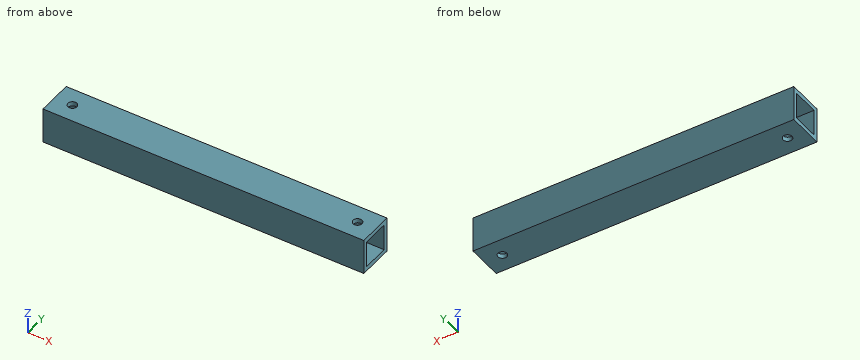
```python
from build123d import *

# Parameters (mm, degrees)
SKETCH1_W           = 228.6
SKETCH1_H           = 25.4
BOSS_EXTRUDE1_DEPTH = 25.4
SKETCH2_W           = 9.525
SKETCH2_H           = 19.040717284
CUT_EXTRUDE1_DEPTH  = 508
SKETCH4_R           = 3.175
CUT_EXTRUDE3_DEPTH  = 508


with BuildPart() as part:
    # Sketch1 → Boss-Extrude1 (new body)
    with BuildSketch(Plane.XY):
        Rectangle(SKETCH1_W, SKETCH1_H)
    extrude(amount=BOSS_EXTRUDE1_DEPTH)

    # Sketch2 → Cut-Extrude1 (cut)
    with BuildSketch(Plane(origin=(114.3, 0, 0), x_dir=(0, 0, -1), z_dir=(1, 0, 0))):
        with Locations((-17.4625, 0)):
            Rectangle(SKETCH2_W, SKETCH2_H)
        with Locations((-7.9375, 0)):
            Rectangle(SKETCH2_W, SKETCH2_H)
    extrude(amount=-CUT_EXTRUDE1_DEPTH, mode=Mode.SUBTRACT)

    # Sketch4 → Cut-Extrude3 (cut)
    with BuildSketch(Plane.XY.offset(25.4)):
        with Locations((-101.6, 0)):
            Circle(SKETCH4_R)
        with Locations((101.6, 0)):
            Circle(SKETCH4_R)
    extrude(amount=-CUT_EXTRUDE3_DEPTH, mode=Mode.SUBTRACT)


solid = part.part
```
Geometry: final body of the model. Coordinates: model frame, mm. Coordinates: 2 decimals unless noted, no trailing zeros. Order: outer loops, then holes, each group sorted by start corner. A loop starts at its lowest first (then second) coordinate and runs counter-clockwise, first axis right, second up. Notation, with made-up numbers: (-8, 74.25) -> (3, 74.25) arc R30 ccw to (3, 104.25) -> close; hole circle Ø4 at (34.25, 20). An arc over 180 degrees is marked (long way). Use CSV: the item, a comma, the result in double quotes.
1) Pin query (flat end, axial travel): pin 1 Ø5.5 at (x, y) = (-101.6, 0) entering from +Z (1 decimal). Return the tip coordinate at first contact, or that it passes through.
Findings:
pin 1,"passes through"
2) Section B-B on y = -5.75. Output: boundary loops of the cut face in (x, z) (3 decimals).
Findings:
outline,"(-114.3, 0) -> (114.3, 0) -> (114.3, 3.175) -> (-114.3, 3.175) -> close; (-114.3, 22.225) -> (114.3, 22.225) -> (114.3, 25.4) -> (-114.3, 25.4) -> close"
3) Section C-C on x = 101.6. Output: boundary loops of the cut face in (y, z) (3 decimals).
Findings:
outline,"(-12.7, 0) -> (-3.175, 0) -> (-3.175, 3.175) -> (-9.52, 3.175) -> (-9.52, 22.225) -> (-3.175, 22.225) -> (-3.175, 25.4) -> (-12.7, 25.4) -> close; (3.175, 0) -> (12.7, 0) -> (12.7, 25.4) -> (3.175, 25.4) -> (3.175, 22.225) -> (9.52, 22.225) -> (9.52, 3.175) -> (3.175, 3.175) -> close"
4) Section D-D on x = 71.5. Output: boundary loops of the cut face in (y, z) (3 decimals).
Findings:
outline,"(-12.7, 0) -> (12.7, 0) -> (12.7, 25.4) -> (-12.7, 25.4) -> close; hole (-9.52, 3.175) -> (9.52, 3.175) -> (9.52, 22.225) -> (-9.52, 22.225) -> close"
5) Section A-A on z = 18.25. Output: boundary loops of the cut face in (x, y), then the cut area to 3 significant figures.
Findings:
outline,"(-114.3, -12.7) -> (114.3, -12.7) -> (114.3, -9.52) -> (-114.3, -9.52) -> close; (-114.3, 9.52) -> (114.3, 9.52) -> (114.3, 12.7) -> (-114.3, 12.7) -> close"
area,"1,450 mm^2"
6) Line query: line 1 (Z direction, x = -58.5, y = 0) (3 decimals); line 2 (Y direction, x = -56.5, z = 13); line 3 (Y direction, x = -101.6, z = 23.75) (3 decimals). Output: solid intervals per line, ascending.
Findings:
line 1,"z = 0 to 3.175, 22.225 to 25.4"
line 2,"y = -12.7 to -9.52, 9.52 to 12.7"
line 3,"y = -12.7 to -3.175, 3.175 to 12.7"
